```python
from build123d import *
from OCP.BRepAlgoAPI import BRepAlgoAPI_Cut
from OCP.TopTools import TopTools_ListOfShape

# Parameters (mm, degrees)
F_7_16_0_4375_DIAMETER_HOLE4_D     = 11.1125
F_7_16_0_4375_DIAMETER_HOLE4_DEPTH = 6.35
F_7_16_0_4375_DIAMETER_HOLE4_TIP   = 3.338531814
CIRPATTERN3_COUNT                  = 6
F_1_2_0_5_DIAMETER_HOLE1_D         = 12.7
F_1_2_0_5_DIAMETER_HOLE1_DEPTH     = 5.08
F_1_2_0_5_DIAMETER_HOLE1_TIP       = 3.815464931


with BuildPart() as part:
    # Sketch1 → Revolve1 (revolve)
    with BuildSketch(Plane.XY, mode=Mode.PRIVATE) as revolve1_sk:
        Polygon((0, 0), (0, 26.570129165), (7.62, 26.570129165), (20.103877155, 17.828824275), (7.62, 0), (7.62, -3.175), (0, -3.175), align=None)
    revolve(revolve1_sk.sketch.rotate(Axis((0, 0, 0), (0, 1, 0)), 90), axis=Axis((0, 0, 0), (0, 1, 0)))

    # 7_16 _0.4375_ Diameter Hole4
    with Locations(Plane(origin=(0.774073223, -3.175, 1.453774394), x_dir=(-1, 0, 0), z_dir=(0, -1, 0))):
        with Locations((0.774073223, 1.453774394)):
            Hole(F_7_16_0_4375_DIAMETER_HOLE4_D / 2, depth=F_7_16_0_4375_DIAMETER_HOLE4_DEPTH)
            with Locations((0, 0, -(F_7_16_0_4375_DIAMETER_HOLE4_DEPTH + F_7_16_0_4375_DIAMETER_HOLE4_TIP / 2))):  # 118° drill point
                Cone(0, F_7_16_0_4375_DIAMETER_HOLE4_D / 2, F_7_16_0_4375_DIAMETER_HOLE4_TIP, mode=Mode.SUBTRACT)


with BuildPart() as f_7_16_0_4375_diameter_hole5_tool:
    # Sketch14 → 7_16 _0.4375_ Diameter Hole5 (revolve)
    with BuildSketch(Plane(origin=(0, 22.123811298, -13.97), x_dir=(0, 0.5735764363510476, 0.8191520442889908), z_dir=(1, 0, 0))):
        Polygon((0, 0), (0, 28.738531814), (5.55625, 25.4), (5.55625, 0), align=None)
    f_7_16_0_4375_diameter_hole5 = revolve(axis=Axis((0, 27.325426779, -17.612210371), (0, -0.8191520442889908, 0.5735764363510476)))


with BuildPart() as part_1:
    add(part.part)

    # 7_16 _0.4375_ Diameter Hole5: cut by f_7_16_0_4375_diameter_hole5_tool, with a tolerance
    f_7_16_0_4375_diameter_hole5_stock = TopTools_ListOfShape()
    f_7_16_0_4375_diameter_hole5_stock.Append(part_1.part.wrapped)
    f_7_16_0_4375_diameter_hole5_tools = TopTools_ListOfShape()
    f_7_16_0_4375_diameter_hole5_tools.Append(f_7_16_0_4375_diameter_hole5_tool.part.wrapped)
    f_7_16_0_4375_diameter_hole5_cut = BRepAlgoAPI_Cut()
    f_7_16_0_4375_diameter_hole5_cut.SetArguments(f_7_16_0_4375_diameter_hole5_stock)
    f_7_16_0_4375_diameter_hole5_cut.SetTools(f_7_16_0_4375_diameter_hole5_tools)
    f_7_16_0_4375_diameter_hole5_cut.SetFuzzyValue(0.00001)
    f_7_16_0_4375_diameter_hole5_cut.Build()
    add(Compound.cast(f_7_16_0_4375_diameter_hole5_cut.Shape()).solids(), mode=Mode.REPLACE)

    # CirPattern3: 7_16 _0.4375_ Diameter Hole5 ×6 about axis
    cirpattern3_axis = Axis((0, 26.570129165, 0), (0, -1, 0))
    for i in range(1, CIRPATTERN3_COUNT):
        add(f_7_16_0_4375_diameter_hole5.rotate(cirpattern3_axis, i * 360 / CIRPATTERN3_COUNT), mode=Mode.SUBTRACT)

    # 1_2 _0.5_ Diameter Hole1
    with Locations(Plane(origin=(0, 26.570129165, 0), x_dir=(1, 0, 0), z_dir=(0, 1, 0))):
        with Locations((0, 0)):
            Hole(F_1_2_0_5_DIAMETER_HOLE1_D / 2, depth=F_1_2_0_5_DIAMETER_HOLE1_DEPTH)
            with Locations((0, 0, -(F_1_2_0_5_DIAMETER_HOLE1_DEPTH + F_1_2_0_5_DIAMETER_HOLE1_TIP / 2))):  # 118° drill point
                Cone(0, F_1_2_0_5_DIAMETER_HOLE1_D / 2, F_1_2_0_5_DIAMETER_HOLE1_TIP, mode=Mode.SUBTRACT)


solid = part_1.part
```
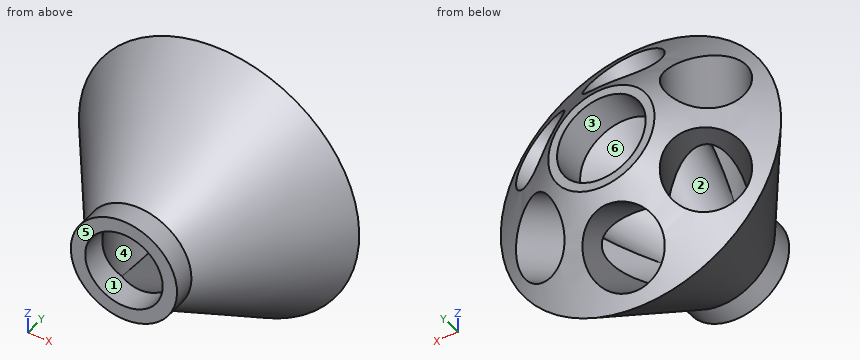
Verification items for the finished model (mm, model axes). Face numbers are marked on the shaded views. A direction names the side the tool comes from. Give positions to 0.01 mm unless a question says otherwise; leave off trailing zeros.
1. Section check A-A, the plane y = 13.75. Count the separate pieces of the cut face and the enclosed holes in it, then the cut area to 3 significant figures.
2. Thickness scan on line 1 (X direction, y = 15.25, z = -1.5); line 2 (X direction, y = 6.75, z = 0.5); line 3 (Z direction, x = 2, y = 21.75). Record the ranges inside material, lowest first.
3. Go/stop test with flat-tipped pins: pin 1 Ø1.5 at (y, z) = (1.5, -5) entering from -X; pin 2 Ø1 at (x, z) = (11.5, 14.5) entering from -Y; pin 3 Ø6 at (x, z) = (1, -11.5) entering from +Y; pin 4 Ø1.5 at (x, y) = (11.5, 2.5) entering from +Z. Record where each tip stops, or that it passes through.
4. Set-up check for the marked faces 1, 2 and 3: record each of +Z, -Z, +X, -X, +Y, -Y from which the full face is reachable in a straight line by a thin tool's end or side.
5. Mould release check, pull along Y, two halves, no side actions. Record for the marked faces 4, 5 and 6: released by +Y, released by -Y, zero draft, split by the parting line, or undercut.
Geometry says:
1. separate pieces: 2
1. enclosed holes: 1
1. area: 365 mm2
2. line 1: x = -18.24 to -12.8, -1.89 to 1.89, 12.8 to 18.24
2. line 2: x = -12.34 to -8.86, 8.86 to 12.34
2. line 3: z = -7.38 to -6.03, 6.03 to 7.38
3. pin 1: stops at x = -7.87
3. pin 2: stops at y = 14.83
3. pin 3: stops at y = 25.92
3. pin 4: passes through
4. face 1: -Y
4. face 2: none
4. face 3: +Y
5. face 4: undercut
5. face 5: released by -Y
5. face 6: released by +Y
